Work out the finished part from the listing and answer in its coordinate system (mm). Give positions to 0.01 mm unless a question says otherwise; leave off trailing zeros. Loops run counter-clockwise (first coordinate to the right, second up) from the corner with the lowest first, then second, coordinate; pieces in that order, holes last. Notation, with made-up numbers: (3, 42.5) - (43, 42.5) arc R23 ccw to (43, 77.5) - close; hole circle Ø8 at (7, 21.5). An arc over 180 degrees is marked (long way). One line per question, with ' | ' between items. Start each with the question number.
1. Find the intervals of material crossed by line 1 (Y direction, x = 0, z = -289); line 2 (X direction, y = 2.5, z = -505.5); line 3 (Y direction, x = -1.5, z = 332), in increasing order.
2. Section C-C (z = 472) is taken. Determine the outline of the cut face in (x, y) (1 decimal), plus the area to 3 significant figures.
3. Section A-A (x = 0) is taken. Determine the outline of the cut face in (y, z).
4. Section D-D (y = 85.5) is taken. Determine the outline of the cut face in (x, z).
5. Each of these flat-tipped pins is pushed along its axis until it touches: pin 1 (6 mm diameter, centred on x = 86, y = -46.5, fed in from +Z); pin 2 (5 mm diameter, centred on x = 44, z = 591.5, fed in from +Y); pin 3 (2 mm diameter, centred on y = 43, z = -414, fed in from -X); pin 4 (12 mm diameter, centred on x = -23, z = -276.5, fed in from -Y). Where does it stop, or does it pass through?
6. For a pull along Y with two mould halves and no side action, classify faces 1 (the face through (-0.428, 111.537, 445.1)), 2 (the face through (97, -31, 800)), 3 (the face through (-21.97, -98.95, -11.2)), 4 (the face through (-23.75, -106.93, -11.2)) as released by +Y, released by -Y, zero draft, split by the parting line, or undercut.
7. Section B-B (y = 0) is taken. Determine the outline of the cut face in (x, z), plus the area to 3 significant figures.
from build123d import *

# Parameters (mm, degrees)
BOSS_EXTRUDE1_DEPTH      = 800
BOSS_EXTRUDE1_DEPTH_BACK = 800
SKETCH3_R                = 109.5375
SKETCH3_R_2              = 101.3587
WRAP2_SECTION_W          = 2
WRAP2_SECTION_H          = 700
WRAP2_ANGLE              = 31.384199665


with BuildPart() as part:
    # Sketch3 → Boss-Extrude1 (new, two sides: drawn at the far end of the back side and taken through both)
    with BuildSketch(Plane.XY.offset(-BOSS_EXTRUDE1_DEPTH_BACK)):
        Circle(SKETCH3_R)
        Circle(SKETCH3_R_2, mode=Mode.SUBTRACT)
    extrude(amount=BOSS_EXTRUDE1_DEPTH + BOSS_EXTRUDE1_DEPTH_BACK)

    # Wrap2 section (on wrap section) → Wrap2 (revolve)
    with BuildSketch(Plane(origin=(0, 0, 0), x_dir=(-0.27046770367687717, 0.9627290487295773, 0), z_dir=(-0.9627290487295773, -0.27046770367687717, 0))):
        with Locations((110.5375, -450)):
            Rectangle(WRAP2_SECTION_W, WRAP2_SECTION_H)
    revolve(axis=Axis((0, 0, 0), (0, 0, -1)), revolution_arc=WRAP2_ANGLE)


solid = part.part
Conclusion:
1) line 1: -109.54 to -101.36, 101.36 to 109.54 | line 2: -109.51 to -101.33, 101.33 to 109.51 | line 3: -109.53 to -101.35, 101.35 to 111.53
2) outline: (-30.2, 107.4) - (-29.6, 105.5) arc R109.5 ccw (long way) to (29.6, 105.5) - (30.2, 107.4) arc R111.5 ccw to start; hole circle Ø202.7 at (0, 0) | area: 5,540 mm²
3) outline: (-109.54, -800) - (-101.36, -800) - (-101.36, 800) - (-109.54, 800) - close; (101.36, -800) - (109.54, -800) - (109.54, 100) - (111.54, 100) - (111.54, 800) - (101.36, 800) - close
4) outline: (-68.47, -800) - (-54.44, -800) - (-54.44, 800) - (-68.47, 800) - close; (54.44, -800) - (68.47, -800) - (68.47, 800) - (54.44, 800) - close
5) pin 1: through | pin 2: y = 101.37 | pin 3: x = -101.17 | pin 4: y = -108.21
6) face 1: released by +Y | face 2: zero draft | face 3: undercut | face 4: split by the parting line
7) outline: (-109.54, -800) - (-101.36, -800) - (-101.36, 800) - (-109.54, 800) - close; (101.36, -800) - (109.54, -800) - (109.54, 800) - (101.36, 800) - close | area: 26,200 mm²
